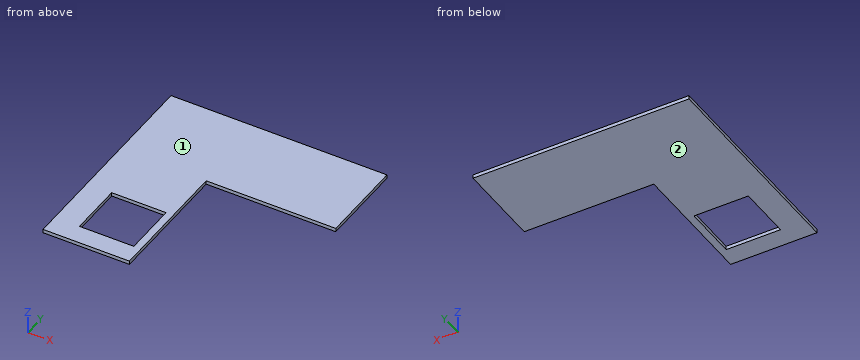
```python
from build123d import *

# Parameters (mm, degrees)
F1_W     = 383.54
F1_H     = 383.54
F2_DEPTH = 25.4


with BuildPart() as f2:
    # F1 (on face) → F2 (new body)
    with BuildSketch(Plane.XY):
        Polygon((914.4, 609.6), (-609.6, 609.6), (-609.6, -914.4), (0, -914.4), (0, 0), (914.4, 0), align=None)
        with Locations((-242.57, -584.2)):
            Rectangle(F1_W, F1_H, mode=Mode.SUBTRACT)
    extrude(amount=F2_DEPTH)


solid = f2.part
```
The model under review builds one solid part; all positions refer to its coordinate system, in mm. Face numbers are marked on the shaded views. Round coordinates to 2 decimals unless told otherwise and drop trailing zeros. Write each loop counter-clockwise with the first axis right and the second up, starting at its lowest first coordinate (ties: lowest second). Pieces come first, ordered by that corner, then holes.
(1) We need section C-C on x = -382.5. Give the boundary of the cut face in (y, z).
(2) Wall thickness on L1, parallel to Y at x = -243, z = 8; L2, parallel to X at y = -421.5, z = 21; L3, parallel to X at y = -103, z = 3.5: over which ranges is each line inside the solid? List them lowest first.
(3) Mouldability with a two-part tool opening along Z and no side actions: class the marked faces 1 and 2 as +Z half, -Z half, draft (parallel to the pull), parting line (faces both ways), or undercut.
(4) We need section B-B on z = 5.25. Give the boundary of the cut face in (x, y).
(5) Insertion check: pin 1 (7.5 mm diameter, centred on x = 509.5, z = 6.5, fed in from -Y); pin 2 (5 mm diameter, centred on y = -34.5, z = 15.5, fed in from +X). Each pin has a flat end and moves straight along its axis. Give the tip position at first contact, or say it passes through.
(6) We need section A-A on y = -535. Give the boundary of the cut face in (x, z).
(7) We need section D-D on x = 741. Give the boundary of the cut face in (y, z), and give its area (3 significant figures).
Findings below:
1. outline: (-914.4, 0) - (-775.97, 0) - (-775.97, 25.4) - (-914.4, 25.4) - close; (-392.43, 0) - (609.6, 0) - (609.6, 25.4) - (-392.43, 25.4) - close
2. L1: y = -914.4 to -775.97, -392.43 to 609.6
2. L2: x = -609.6 to -434.34, -50.8 to 0
2. L3: x = -609.6 to 0
3. face 1: +Z half
3. face 2: -Z half
4. outline: (-609.6, -914.4) - (0, -914.4) - (0, 0) - (914.4, 0) - (914.4, 609.6) - (-609.6, 609.6) - close; hole (-434.34, -775.97) - (-50.8, -775.97) - (-50.8, -392.43) - (-434.34, -392.43) - close
5. pin 1: stops at y = 0
5. pin 2: stops at x = 0
6. outline: (-609.6, 0) - (-434.34, 0) - (-434.34, 25.4) - (-609.6, 25.4) - close; (-50.8, 0) - (0, 0) - (0, 25.4) - (-50.8, 25.4) - close
7. outline: (0, 0) - (609.6, 0) - (609.6, 25.4) - (0, 25.4) - close
7. area: 15,500 mm2
